```python
from build123d import *

# Parameters (mm, degrees)
F0_R     = 25
F1_DEPTH = 10.8
F2_SIZE2 = 1.8
F2_SIZE  = 5.6
F3_R     = 2.5
F4_DEPTH = 6
F5_SIZE  = 2.2
F3_R_2   = 6.5
F6_DEPTH = 10.801
F8_DEPTH = 4.2


with BuildPart() as f1:
    # F0 (on Top) → F1 (new body)
    with BuildSketch(Plane.XY):
        Circle(F0_R)
    extrude(amount=F1_DEPTH)

    # F2
    f2_edges = [f1.edges().sort_by_distance(p)[0] for p in [
        (-25, 0, 10.8),
    ]]
    f2_side = f1.faces().sort_by_distance((0, 0, 10.8))[0]
    chamfer(f2_edges, length=F2_SIZE, length2=F2_SIZE2, reference=f2_side)

    # F3 (on face) → F4 (join)
    with BuildSketch(Plane.XY.offset(10.8)):
        with Locations((-10.9456407546, 8.728857226)):
            Circle(F3_R)
        with Locations((0, 14)):
            Circle(F3_R)
        with Locations((10.9456407546, 8.728857226)):
            Circle(F3_R)
        with Locations((13.6489907705, -3.1152930754)):
            Circle(F3_R)
        with Locations((6.0743723476, -12.6135641506)):
            Circle(F3_R)
        with Locations((-6.0743723476, -12.6135641506)):
            Circle(F3_R)
        with Locations((-13.6489907705, -3.1152930754)):
            Circle(F3_R)
    extrude(amount=F4_DEPTH)

    # F5
    f5_edges = [f1.edges().sort_by_distance(p)[0] for p in [
        (-2.5, 14, 16.8),
        (8.445641, 8.728857, 16.8),
        (11.148991, -3.115293, 16.8),
        (3.574372, -12.613564, 16.8),
        (-8.574372, -12.613564, 16.8),
        (-16.148991, -3.115293, 16.8),
        (-13.445641, 8.728857, 16.8),
    ]]
    chamfer(f5_edges, length=F5_SIZE)

    # F3 (on face) → F6 (cut, through all)
    with BuildSketch(Plane.XY.offset(10.8)):
        Circle(F3_R_2)
    extrude(amount=-F6_DEPTH, mode=Mode.SUBTRACT)

    # F7 (on face) → F8 (cut)
    with BuildSketch(Plane(origin=(0, 0, 0), x_dir=(1, 0, 0), z_dir=(0, 0, -1))):
        with BuildLine():
            Line((4.6488008791, 9.9693856574), (9.72022002, 20.8450791018))
            ThreePointArc((9.72022002, 20.8450791018), (4.9781111206, 22.4548081638), (0, 23))
            Line((0, 23), (0, 11))
            ThreePointArc((0, 11), (2.3808357533, 10.7392560783), (4.6488008791, 9.9693856574))
        make_face()
        with BuildLine():
            Line((9.9693856574, 4.6488008791), (20.8450791018, 9.72022002))
            ThreePointArc((20.8450791018, 9.72022002), (18.2471268267, 14.0015128672), (14.7841150228, 17.6190221917))
            Line((14.7841150228, 17.6190221917), (7.0706637066, 8.4264888743))
            ThreePointArc((7.0706637066, 8.4264888743), (8.7268867432, 6.6963757191), (9.9693856574, 4.6488008791))
        make_face()
        with BuildLine():
            ThreePointArc((22.2162940046, -5.9528380374), (22.8032318116, -3.0021024211), (23, 0))
            ThreePointArc((23, 0), (22.9124780561, 2.0045820832), (22.6505783193, 3.9939080863))
            Line((22.6505783193, 3.9939080863), (10.8328852831, 1.9101299543))
            ThreePointArc((10.8328852831, 1.9101299543), (10.958141679, 0.9587131702), (11, 0))
            ThreePointArc((11, 0), (10.9058934751, -1.4357881144), (10.6251840892, -2.8470094961))
            Line((10.6251840892, -2.8470094961), (22.2162940046, -5.9528380374))
        make_face()
        with BuildLine():
            ThreePointArc((13.1922580361, -18.8404970186), (16.9573787466, -15.5385747752), (19.918584287, -11.5))
            Line((19.918584287, -11.5), (9.5262794416, -5.5))
            ThreePointArc((9.5262794416, -5.5), (8.1100507049, -7.4314922838), (6.3093407999, -9.0106724872))
            Line((6.3093407999, -9.0106724872), (13.1922580361, -18.8404970186))
        make_face()
        with BuildLine():
            ThreePointArc((-2.0045820832, -22.9124780561), (3.0021024211, -22.8032318116), (7.8664632965, -21.6129302781))
            Line((7.8664632965, -21.6129302781), (3.7622215766, -10.3366188286))
            ThreePointArc((3.7622215766, -10.3366188286), (1.4357881144, -10.9058934751), (-0.9587131702, -10.958141679))
            Line((-0.9587131702, -10.958141679), (-2.0045820832, -22.9124780561))
        make_face()
        with BuildLine():
            Line((-7.8664632965, -21.6129302781), (-3.7622215766, -10.3366188286))
            ThreePointArc((-3.7622215766, -10.3366188286), (-5.9102956918, -9.2773059039), (-7.7781745931, -7.7781745931))
            Line((-7.7781745931, -7.7781745931), (-16.2634559673, -16.2634559673))
            ThreePointArc((-16.2634559673, -16.2634559673), (-12.357890992, -19.3980032537), (-7.8664632965, -21.6129302781))
        make_face()
        with BuildLine():
            Line((-19.918584287, -11.5), (-9.5262794416, -5.5))
            ThreePointArc((-9.5262794416, -5.5), (-10.4908864582, -3.3077637945), (-10.958141679, -0.9587131702))
            Line((-10.958141679, -0.9587131702), (-22.9124780561, -2.0045820832))
            ThreePointArc((-22.9124780561, -2.0045820832), (-21.9354898672, -6.9162333886), (-19.918584287, -11.5))
        make_face()
        with BuildLine():
            Line((-22.6505783193, 3.9939080863), (-10.8328852831, 1.9101299543))
            ThreePointArc((-10.8328852831, 1.9101299543), (-10.1626748576, 4.209517756), (-9.0106724872, 6.3093407999))
            Line((-9.0106724872, 6.3093407999), (-18.8404970186, 13.1922580361))
            ThreePointArc((-18.8404970186, 13.1922580361), (-21.2492292478, 8.8017189444), (-22.6505783193, 3.9939080863))
        make_face()
        with BuildLine():
            Line((-2.8470094961, 10.6251840892), (-5.9528380374, 22.2162940046))
            ThreePointArc((-5.9528380374, 22.2162940046), (-10.6202181044, 20.4012491631), (-14.7841150228, 17.6190221917))
            Line((-14.7841150228, 17.6190221917), (-7.0706637066, 8.4264888743))
            ThreePointArc((-7.0706637066, 8.4264888743), (-5.0792347456, 9.757119165), (-2.8470094961, 10.6251840892))
        make_face()
    extrude(amount=-F8_DEPTH, mode=Mode.SUBTRACT)


solid = f1.part
```
CAD build for the part. Positions are in the model's coordinates, mm. A direction names the side the tool comes from. Coordinates: 2 decimals unless noted, no trailing zeros. Order: outer loops, then holes, each group sorted by start corner. A loop starts at its lowest first (then second) coordinate and runs counter-clockwise, first axis right, second up. Notation, with made-up numbers: (62, 2) -> (98, 2) arc R11 cw to (98, 20) -> close; hole circle Ø11 at (75.25, -2.5). An arc over 180 degrees is marked (long way). Use one line per item in the form item = value. Start each with the question number.
1) Drop flat-ended pins along their axis: pin 1 (10 mm diameter, centred on x = -11, z = 7.5, fed in from +Y); pin 2 (1 mm diameter, centred on x = 1.5, y = 7.5, fed in from +Z); pin 3 (1 mm diameter, centred on x = -12, z = 3.5, fed in from +Y). Give the stop position or say it passes through.
2) Drill centre lines: L1, parallel to X at y = 21, z = 2; L2, parallel to Y at x = -10, z = 7.5; L3, parallel to X at y = -1.5, z = 5.75. Where is each one in solid material? Low to high. Write a range as [from, to].
3) Band-saw the part on A-A on z = 7. Give the cut face in (x, y), then the cut area to 3 significant figures.
4) Pull direction Y, two halves, no side cores. Call faces 3 (the flat face through (-9, -15, 4.2)), 4 (the cylindrical face through (-5.158, -3.955, 5.476)): +Y half, -Y half, draft (parallel to the pull), parting line (faces both ways), or undercut.
5) Tool access for faces 1 (the flat face through (-13.857, -9.703, 2.071)), 2 (the cylindrical face through (-8.56, 9.48, 12.67)): list every direction of +Z, -Z, +X, -X, +Y, -Y with a clear straight run to the whole face (end or side of a thin tool).
Entries:
q1.pin_1 = 24.27
q1.pin_2 = 10.8
q1.pin_3 = 22.2
q2.L1 = [-13.56, -9.38], [-7.64, -1.84], [7.64, 13.56]
q2.L2 = [-22.91, 22.91]
q2.L3 = [-24.95, -6.32], [6.32, 24.95]
q3.outline = circle Ø50 at (0, 0); hole circle Ø13 at (0, 0)
q3.area = 1,830 mm2
q4.face_3 = undercut
q4.face_4 = undercut
q5.face_1 = -Z
q5.face_2 = +Z
